from build123d import *

# Parameters (mm, degrees)
SKETCH_W     = 21
SKETCH_H     = 10
PAD_DEPTH    = 0.8
SKETCH001_W  = 8
SKETCH001_H  = 1.2
PAD001_DEPTH = 11
SKETCH002_W  = 8
SKETCH002_H  = 1.2
PAD002_DEPTH = 11
SKETCH003_R  = 0.25
POCKET_DEPTH = 3
SKETCH004_R  = 1.5
HOLE_DEPTH   = 1.601


with BuildPart() as part:
    # Sketch → Pad (new body)
    with BuildSketch(Plane.XY):
        Rectangle(SKETCH_W, SKETCH_H)
    extrude(amount=PAD_DEPTH)

    # Sketch001 (on Face1 of Pad) → Pad001 (join)
    with BuildSketch(Plane(origin=(0, 5, 0), x_dir=(-1, 0, 0), z_dir=(0, 1, 0))):
        with Locations((0, -0.2)):
            Rectangle(SKETCH001_W, SKETCH001_H)
    extrude(amount=PAD001_DEPTH)

    # Sketch002 (on Face1 of Pad001) → Pad002 (join)
    with BuildSketch(Plane(origin=(0, 5, 0), x_dir=(-1, 0, 0), z_dir=(0, 1, 0))):
        with Locations((0, 1)):
            Rectangle(SKETCH002_W, SKETCH002_H)
    extrude(amount=PAD002_DEPTH)

    # Sketch003 (on Face5 of Pad002) → Pocket (cut)
    with BuildSketch(Plane.XY.offset(0.8)):
        with Locations((-9, -3.55)):
            Circle(SKETCH003_R)
        with Locations((-7.5, -3.55)):
            Circle(SKETCH003_R)
        with Locations((-3, -3.55)):
            Circle(SKETCH003_R)
        with Locations((4.5, -3.55)):
            Circle(SKETCH003_R)
        with Locations((9, -3.55)):
            Circle(SKETCH003_R)
    extrude(amount=-POCKET_DEPTH, mode=Mode.SUBTRACT)

    # Sketch004 (on Face5 of Pocket) → Hole (cut, through all)
    with BuildSketch(Plane.XY.offset(0.8)):
        with Locations((-8, 2.5)):
            Circle(SKETCH004_R)
        with Locations((8, 2.5)):
            Circle(SKETCH004_R)
    extrude(amount=-HOLE_DEPTH, mode=Mode.SUBTRACT)


solid = part.part
Work out the finished part from the listing and answer in its coordinate system (mm). A direction names the side the tool comes from. Give positions to 0.01 mm unless a question says otherwise; leave off trailing zeros. Loops run counter-clockwise (first coordinate to the right, second up) from the corner with the lowest first, then second, coordinate; pieces in that order, holes last. Notation, with made-up numbers: (37, 15.25) -> (82, 15.25) arc R29 cw to (82, 37.25) -> close; hole circle Ø3 at (-17, -5). An arc over 180 degrees is marked (long way). Use a Markdown table: item, result. Add a question column.
1. Determine the mould class of faces 4 (the flat face through (0, 0, 0.8)), 5 (the flat face through (0, 16, 0)), 6 (the cylindrical face through (-9.2, 1.6, 0.4)) for opening direction Y: released by +Y, released by -Y, zero draft, split by the parting line, or undercut.
2. Section C-C on y = -3.55 is taken. Determine the outline of the cut face in (x, z).
3. For faces 1 (the flat face through (-4, 10, 0)), 2 (the flat face through (0, 0, 0)), 3 (the flat face through (4, 10, 0)), determine the directions among +Z, -Z, +X, -X, +Y, -Y from which every point of the face is accessible in a straight line to the end or side of a thin tool.
4. Flat-ended cylindrical pins translate along their axes: pin 1 Ø8 at (x, y) = (-8, 1.5) entering from -Z; pin 2 Ø1 at (x, z) = (6, 1) entering from +Y; pin 3 Ø3.5 at (x, y) = (8, 2.5) entering from +Z; pin 4 Ø2.5 at (x, y) = (-8, 2.5) entering from +Z. Find the tip coordinate at first contact, or state that the pin passes through.
5. Find the intervals of material crossed by probe 1 along Y at (x, z) = (4.5, 0.3); probe 2 along Y at (x, z) = (-8, 0.65); probe 3 along Y at (x, z) = (-7.5, 0.25), in increasing order.
6. Section A-A on x = 8 is taken. Determine the outline of the cut face in (y, z), and give its area (3 significant figures).
7. Section D-D on x = -7.5 is taken. Determine the outline of the cut face in (y, z), and give its area (3 significant figures).
8. Section B-B on y = 2.5 is taken. Determine the outline of the cut face in (x, z).
Results below:
| question | item | result |
|---|---|---|
| 1 | face 4 | zero draft |
| 1 | face 5 | released by +Y |
| 1 | face 6 | undercut |
| 2 | outline | (-10.5, 0) -> (-9.25, 0) -> (-9.25, 0.8) -> (-10.5, 0.8) -> close; (-8.75, 0) -> (-7.75, 0) -> (-7.75, 0.8) -> (-8.75, 0.8) -> close; (-7.25, 0) -> (-3.25, 0) -> (-3.25, 0.8) -> (-7.25, 0.8) -> close; (-2.75, 0) -> (4.25, 0) -> (4.25, 0.8) -> (-2.75, 0.8) -> close; (4.75, 0) -> (8.75, 0) -> (8.75, 0.8) -> (4.75, 0.8) -> close; (9.25, 0) -> (10.5, 0) -> (10.5, 0.8) -> (9.25, 0.8) -> close |
| 3 | face 1 | +Z, -Z, -X, +Y |
| 3 | face 2 | -Z, +X, -X, -Y |
| 3 | face 3 | +Z, -Z, +X, +Y |
| 4 | pin 1 | stops at z = 0 |
| 4 | pin 2 | stops at y = 5 |
| 4 | pin 3 | stops at z = 0.8 |
| 4 | pin 4 | passes through |
| 5 | probe 1 | y = -5 to -3.8, -3.3 to 5 |
| 5 | probe 2 | y = -5 to 1, 4 to 5 |
| 5 | probe 3 | y = -5 to -3.8, -3.3 to 1.09, 3.91 to 5 |
| 6 | outline | (-5, 0) -> (1, 0) -> (1, 0.8) -> (-5, 0.8) -> close; (4, 0) -> (5, 0) -> (5, 0.8) -> (4, 0.8) -> close |
| 6 | area | 5.60 mm^2 |
| 7 | outline | (-5, 0) -> (-3.8, 0) -> (-3.8, 0.8) -> (-5, 0.8) -> close; (-3.3, 0) -> (1.09, 0) -> (1.09, 0.8) -> (-3.3, 0.8) -> close; (3.91, 0) -> (5, 0) -> (5, 0.8) -> (3.91, 0.8) -> close |
| 7 | area | 5.34 mm^2 |
| 8 | outline | (-10.5, 0) -> (-9.5, 0) -> (-9.5, 0.8) -> (-10.5, 0.8) -> close; (-6.5, 0) -> (6.5, 0) -> (6.5, 0.8) -> (-6.5, 0.8) -> close; (9.5, 0) -> (10.5, 0) -> (10.5, 0.8) -> (9.5, 0.8) -> close |
